Print and shaded views of the part. All mm, measured from the part's lowest x, y and z. A direction names the side the tool comes from. Round coordinates to 2 decimals unless told otherwise and drop trailing zeros. Loops run counter-clockwise (first coordinate to the right, second up) from the corner with the lowest first, then second, coordinate; pieces in that order, holes last. Notation, with made-up numbers: (14.25, -4.75) -> (69.25, -4.75) arc R18 ccw to (69.25, 24.25) -> close; hole circle Ø6 at (77.5, -25). An arc over 180 degrees is marked (long way). Use a Markdown table: item, result.
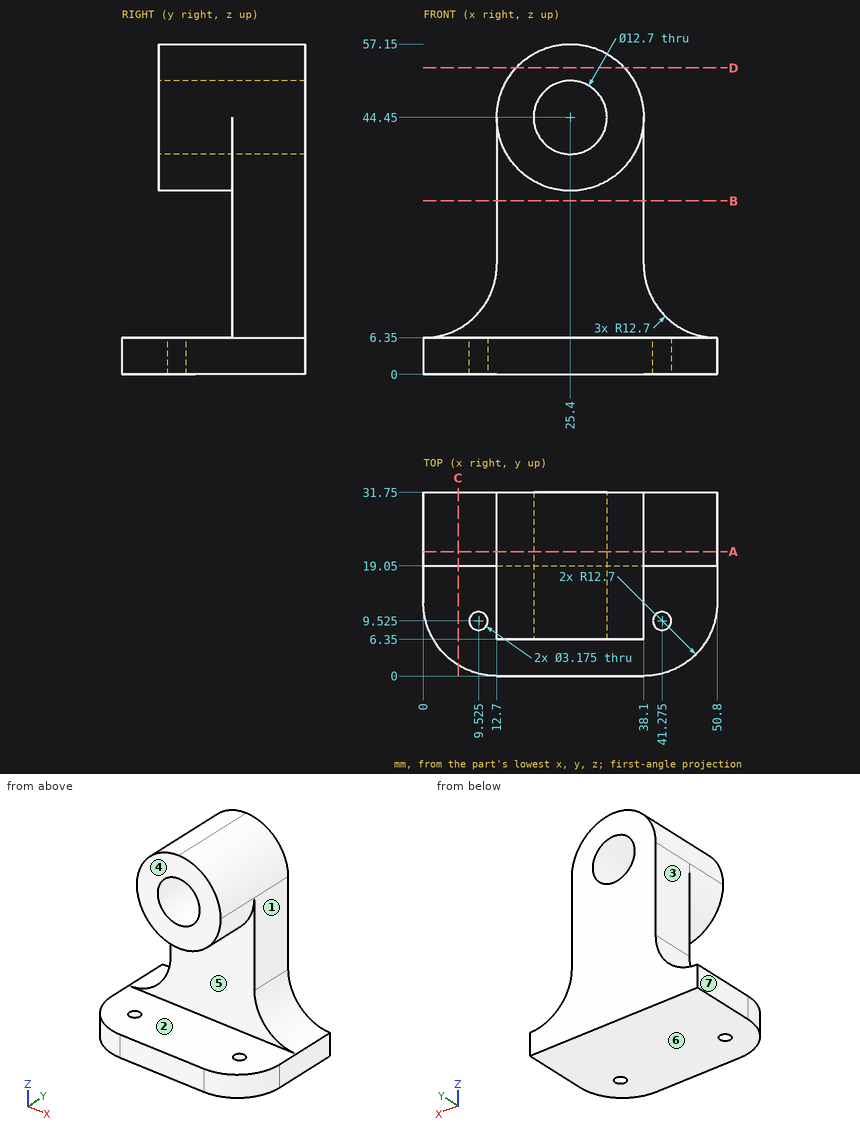
Q1. Band-saw the part on C-C, the plane x = 6. Give the cut face in (y, z), plus the area to 3 significant figures.
Results list:
| item | result |
|---|---|
| outline | (1.91, 0) -> (31.75, 0) -> (31.75, 7.86) -> (19.05, 7.86) -> (19.05, 6.35) -> (1.91, 6.35) -> close |
| area | 209 mm² |
Q2. Band-saw the part on D-D, the plane z = 53. Give the cut face in (x, y).
Results list:
| item | result |
|---|---|
| outline | (16.01, 6.35) -> (34.79, 6.35) -> (34.79, 31.75) -> (16.01, 31.75) -> close |
Q3. Band-saw the part on B-B, the plane z = 30. Give the cut face in (x, y), plus the area to 3 significant figures.
Results list:
| item | result |
|---|---|
| outline | (12.7, 19.05) -> (38.1, 19.05) -> (38.1, 31.75) -> (12.7, 31.75) -> close |
| area | 323 mm² |
Q4. Flat gauge pins, fed straight in: pin 1 (12 mm diameter, centred on x = 27.5, z = 20.5, fed in from -Y); pin 2 (2 mm diameter, centred on x = 33, z = 38, fed in from -Y); pin 3 (1 mm diameter, centred on x = 23.5, y = 21.5, fed in from +Z). Where does each tip first touch, or does it go through?
Results list:
| item | result |
|---|---|
| pin 1 | stops at y = 19.05 |
| pin 2 | stops at y = 6.35 |
| pin 3 | stops at z = 57.07 |
Q5. Drill centre lines: L1, parallel to Y at x = 18, z = 35; L2, parallel to Y at x = 23.5, z = 14; L3, parallel to Z at x = 39, y = 5. Where is each one in solid material? Low to high. Write a range as from..to.
Results list:
| item | result |
|---|---|
| L1 | y = 6.35..31.75 |
| L2 | y = 19.05..31.75 |
| L3 | z = 0..6.35 |
Q6. Band-saw the part on A-A, the plane y = 21.5. Give the cut face in (x, z), plus the area to 3 significant figures.
Results list:
| item | result |
|---|---|
| outline | (0, 0) -> (50.8, 0) -> (50.8, 6.35) arc R12.7 cw to (38.1, 19.05) -> (38.1, 44.45) arc R12.7 ccw to (12.7, 44.45) -> (12.7, 19.05) arc R12.7 cw to (0, 6.35) -> close; hole circle Ø12.7 at (25.4, 44.45) |
| area | 1,490 mm² |
Q7. Tool access for the marked faces 1, 2, 3 and 4: list every direction of +Z, -Z, +X, -X, +Y, -Y with a clear straight run to the whole face (end or side of a thin tool).
Results list:
| item | result |
|---|---|
| face 1 | +Z, +X, +Y, -Y |
| face 2 | +X, -X, -Y |
| face 3 | +Z, -X, +Y, -Y |
| face 4 | +Z, +X, -X, -Y |
Q8. Pull direction Z, two halves, no side cores. Call the marked faces 5, 6 and 7: released by +Z, released by -Z, zero draft, split by the parting line, or undercut.
Results list:
| item | result |
|---|---|
| face 5 | undercut |
| face 6 | released by -Z |
| face 7 | zero draft |
